Autodesk Inventor part; units mm, degrees
ref_plane "YZ Plane" through (0, 0, 0) normal (1, 0, 0) x (0, 1, 0)
ref_plane "XZ Plane" through (0, 0, 0) normal (0, 1, 0) x (-1, 0, 0)
ref_plane "XY Plane" through (0, 0, 0) normal (0, 0, 1) x (1, 0, 0)
sketch "Sketch1" plane through (0, 0, 0) normal (0, 0, 1) x (1, 0, 0)
  line L0 (0, 0) -> (31.75, 0)
  line L1 (31.75, 0) -> (31.75, 6.35)
  line L2 (31.75, 25.4) -> (28.575, 25.4) construction
  line L3 (0, 25.4) -> (0, 6.35) construction
  line L4 (0, 6.35) -> (3.175, 6.35)
  line L5 (3.175, 6.35) -> (3.175, 25.4)
  line L6 (28.575, 25.4) -> (28.575, 6.35)
  line L7 (28.575, 6.35) -> (31.75, 6.35)
  line L8 (0, 6.35) -> (0, 0)
  line L9 (3.175, 25.4) -> (0, 25.4) construction
  line L10 (28.575, 25.4) -> (3.175, 25.4)
  line L11 (31.75, 6.35) -> (31.75, 25.4) construction
  dimension "d0" = 31.75
  dimension "d1" = 25.4
  dimension "d2" = 6.35
  dimension "d3" = 3.175
extrude "Extrusion1" add sketch "Sketch1" along normal blind 155.575
sketch "Sketch2" plane through (3.175, 25.4, 0) normal (0, 1, 0) x (1, 0, 0)
  line L0 (0, -155.575) -> (25.4, -155.575)
  line L1 (25.4, 0) -> (25.4, -155.575)
  line L2 (25.4, 0) -> (0, 0)
  line L3 (0, 0) -> (0, -155.575)
  point P0 (-3.175, 0)
  point P1 (12.7, -142.875)
  point P2 (12.7, -12.7)
  dimension "d6" = 12.7
  dimension "d7" = 12.7
  dimension "d8" = 12.7
  dimension "d9" = 12.7
hole "Hole1" at (15.875, 25.4, 142.875) at (15.875, 25.4, 12.7) direction (0, -1, 0) diameter 6.35 end through all counterbore diameter 9.525 counterbore depth 6.35
properties part number "8 ball plastic slider 2"
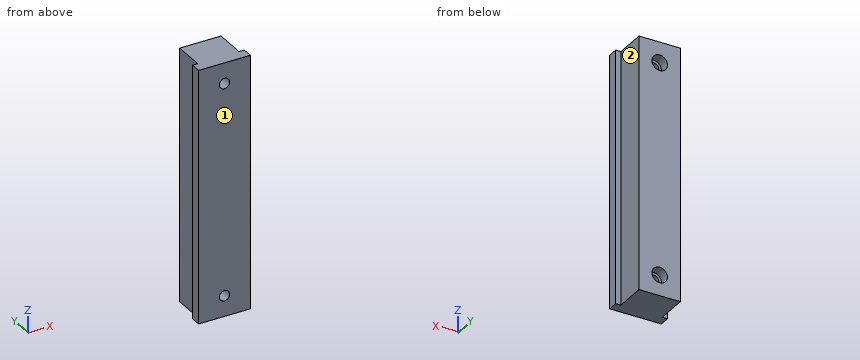
Geometry check sheet. Reference: the model listing, model coordinates, mm. Face numbers are marked on the shaded views. A direction names the side the tool comes from. Coordinates: 2 decimals unless noted, no trailing zeros. Order: outer loops, then holes, each group sorted by start corner. A loop starts at its lowest first (then second) coordinate and runs counter-clockwise, first axis right, second up. Notation, with made-up numbers: (45.25, -12.5) - (90.25, -12.5) arc R6 cw to (90.25, -8.5) - close; hole circle Ø6 at (-32, 39). An arc over 180 degrees is marked (long way). Answer as a JSON object with one key per item and string values. Group by question number.
Item 1: Depth check by flat-ended pin: pin 1 Ø5.5 at (x, z) = (15.875, 142.875) entering from +Y; pin 2 Ø5.5 at (y, z) = (18, 79.5) entering from -X (3 decimals); pin 3 Ø9.5 at (y, z) = (14, 115.5) entering from +X (3 decimals); pin 4 Ø1.6 at (x, z) = (30.5, 71.5) entering from +Y. Enter the tip coordinate at first touch or a pass-through.
Item 2: Sectioned sample at C-C, the plane z = 31. Record the cut outline in (x, y) (3 decimals), and give its area (3 significant figures).
Item 3: Tool access check on the marked faces 1 and 2. Record the directions out of +Z, -Z, +X, -X, +Y, -Y that give a thin tool (end or side, any length) a straight path to the whole face; none if there is none.
Item 4: Sectioned sample at B-B, the plane y = 17.25. Record the cut outline in (x, z) (3 decimals).
Item 5: Scan lines: probe 1 along X at (y, z) = (23.5, 12.7) (1 decimal); probe 2 along Z at (x, y) = (18.5, 4.25) (3 decimals); probe 3 along Z at (x, y) = (14, 8) (3 decimals). Record each from-to range of solid material in increasing order.
Resolved:
{
 "1": {"pin 1": "through", "pin 2": "x = 3.175", "pin 3": "x = 28.575", "pin 4": "y = 6.35"},
 "2": {"outline": "(0, 0) - (31.75, 0) - (31.75, 6.35) - (28.575, 6.35) - (28.575, 25.4) - (3.175, 25.4) - (3.175, 6.35) - (0, 6.35) - close", "area": "685 mm^2"},
 "3": {"face 1": "+Z, -Z, +X, -X, -Y", "face 2": "+Z, -Z, +X, +Y"},
 "4": {"outline": "(3.175, 0) - (28.575, 0) - (28.575, 155.575) - (3.175, 155.575) - close; hole circle Ø6.35 at (15.875, 12.7); hole circle Ø6.35 at (15.875, 142.875)"},
 "5": {"probe 1": "3.2 to 11.1, 20.6 to 28.6", "probe 2": "0 to 10.914, 14.486 to 141.089, 144.661 to 155.575", "probe 3": "0 to 10.138, 15.262 to 140.313, 145.437 to 155.575"}
}
